Autodesk Inventor part; units mm, degrees
ref_plane "YZ Plane" through (0, 0, 0) normal (1, 0, 0) x (0, 1, 0)
ref_plane "XZ Plane" through (0, 0, 0) normal (0, 1, 0) x (-1, 0, 0)
ref_plane "XY Plane" through (0, 0, 0) normal (0, 0, 1) x (1, 0, 0)
sketch "Sketch3" plane through (0, 0, 0) normal (0, 0, 1) x (1, 0, 0)
  line L0 (-50, 45) -> (50, 45)
  line L1 (50, 45) -> (50, -45)
  line L2 (50, -45) -> (-50, -45)
  line L3 (-50, -45) -> (-50, 45)
  line L4 (-50, 45) -> (50, -45) construction
  line L5 (50, 45) -> (-50, -45) construction
  point P0 (0, 0)
  dimension "d4" = 100
  dimension "d5" = 90
extrude "Extrusion2" add sketch "Sketch3" along normal blind 4
sketch "Sketch4" plane through (0, 0, 4) normal (0, 0, 1) x (1, 0, 0)
  point P0 (0, 0)
sketch "Sketch5" plane through (0, 0, 4) normal (0, 0, 1) x (1, 0, 0)
  line L0 (50, 45) -> (-50, 45)
  line L1 (50, 45) -> (-50, 45)
  line L2 (-50, 45) -> (-50, 41)
  line L3 (-50, 41) -> (50, 41)
  line L4 (50, 41) -> (50, 45)
  point P0 (0, 0)
  dimension "d8" = 4
  dimension "d9" = 100
extrude "Extrusion3" add sketch "Sketch5" against normal blind 50
sketch "Sketch6" plane through (0, 0, 4) normal (0, 0, 1) x (1, 0, 0)
  line L0 (18, -31.18) -> (-18, -31.18)
  line L1 (-18, -31.18) -> (-18, 31.18)
  line L2 (-18, 31.18) -> (18, 31.18)
  line L3 (18, 31.18) -> (18, -31.18)
  line L4 (18, -31.18) -> (-18, 31.18) construction
  line L5 (-18, -31.18) -> (18, 31.18) construction
  circle A0 centre (-18, 31.18) radius 1.75
  circle A1 centre (18, 31.18) radius 1.75
  circle A2 centre (-18, -31.18) radius 1.75
  circle A3 centre (18, -31.18) radius 1.75
  point P0 (0, 0)
  dimension "d12" = 36
  dimension "d13" = 62.36
  dimension "d14" = 3.5
  dimension "d15" = 3.5
  dimension "d16" = 3.5
  dimension "d17" = 3.5
extrude "Extrusion4" cut sketch "Sketch6" against normal blind 50 contours A2 L1 L0 | L0 L1 A2 | A3 L3 L0 | L0 L3 A3 | A0 L2 L1 | L1 L2 A0 | A1 L2 L3 | L3 L2 A1
sketch "Sketch7" plane through (0, 0, 4) normal (0, 0, 1) x (1, 0, 0)
  line L0 (31.18, -18) -> (-31.18, -18)
  line L1 (-31.18, -18) -> (-31.18, 18)
  line L2 (-31.18, 18) -> (31.18, 18)
  line L3 (31.18, 18) -> (31.18, -18)
  line L4 (31.18, -18) -> (-31.18, 18) construction
  line L5 (-31.18, -18) -> (31.18, 18) construction
  circle A0 centre (-31.18, 18) radius 1.75
  circle A1 centre (31.18, 18) radius 1.75
  circle A2 centre (-31.18, -18) radius 1.75
  circle A3 centre (31.18, -18) radius 1.75
  point P0 (0, 0)
  dimension "d20" = 62.36
  dimension "d21" = 36
  dimension "d22" = 3.5
  dimension "d23" = 3.5
  dimension "d24" = 3.5
  dimension "d25" = 3.5
extrude "Extrusion5" cut sketch "Sketch7" against normal blind 50 contours A2 L1 L0 | L0 L1 A2 | A3 L3 L0 | L0 L3 A3 | A0 L2 L1 | L1 L2 A0 | A1 L2 L3 | L3 L2 A1
sketch "Sketch8" plane through (0, 0, 4) normal (0, 0, 1) x (1, 0, 0)
  circle A0 centre (0, 0) radius 25
  dimension "d28" = 50
extrude "Extrusion6" cut sketch "Sketch8" against normal blind 43.6625
sketch "Sketch9" plane through (-50, 45, 4) normal (0, 1, 0) x (1, 0, 0)
  line L0 (0, 50) -> (0, 0)
  line L1 (100, 0) -> (0, 0)
  line L2 (0, 0) -> (38, 0)
  line L3 (38, 0) -> (38, 7)
  line L4 (38, 7) -> (0, 7)
  line L5 (0, 7) -> (0, 0)
  circle A0 centre (38, 7) radius 1.75
  line L6 (0, 0) -> (38, 0)
  line L7 (38, 0) -> (38, 25)
  line L8 (38, 25) -> (0, 25)
  line L9 (0, 25) -> (0, 0)
  circle A1 centre (38, 25) radius 1.75
  point P0 (50, 4)
  dimension "d31" = 38
  dimension "d32" = 7
  dimension "d36" = 3.5
  dimension "d39" = 25
  dimension "d40" = 3.5
sketch "Sketch10" plane through (-50, 45, 4) normal (0, 1, 0) x (1, 0, 0)
  line L0 (100, 4) -> (100, 0)
  line L1 (100, 0) -> (0, 0)
  line L2 (100, 0) -> (62, 0)
  line L3 (62, 0) -> (62, 7)
  line L4 (62, 7) -> (100, 7)
  line L5 (100, 7) -> (100, 0)
  circle A0 centre (62, 7) radius 1.75
  line L6 (100, 0) -> (62, 0)
  line L7 (62, 0) -> (62, 25)
  line L8 (62, 25) -> (100, 25)
  line L9 (100, 25) -> (100, 0)
  line L10 (75, 0) -> (25, 0)
  circle A1 centre (62, 25) radius 1.75
  point P0 (50, 4)
  dimension "d33" = 38
  dimension "d34" = 7
  dimension "d35" = 3.5
  dimension "d37" = 25
  dimension "d38" = 3.5
sketch "Sketch11" plane through (-50, 45, 4) normal (0, 1, 0) x (1, 0, 0)
  point P0 (50, 4)
extrude "Extrusion7" cut sketch "Sketch9" against normal blind 43.6625 contours A1 L7 L8 | L8 L7 A1 | A0 L7 L4 | L4 L3 A0 | L7 A0 L3
extrude "Extrusion8" cut sketch "Sketch10" against normal blind 43.6625 contours A0 L3 L4 | L4 L7 A0 | L3 A0 L7 | A1 L7 L8 | L8 L7 A1
sketch "Sketch12" plane through (-50, 45, 4) normal (0, 1, 0) x (1, 0, 0)
  line L0 (0, 0) -> (100, 0)
  line L1 (0, 0) -> (10, 0)
  line L2 (10, 0) -> (10, 7)
  line L3 (10, 7) -> (0, 7)
  line L4 (0, 7) -> (0, 0)
  line L5 (100, 0) -> (0, 0)
  line L6 (0, 0) -> (10, 0)
  line L7 (10, 0) -> (10, 25)
  line L8 (10, 25) -> (0, 25)
  line L9 (0, 25) -> (0, 0)
  circle A0 centre (10, 7) radius 1.75
  circle A1 centre (10, 25) radius 1.75
  point P0 (50, 4)
  dimension "d45" = 10
  dimension "d46" = 7
  dimension "d47" = 25
  dimension "d48" = 3.5
  dimension "d49" = 3.5
extrude "Extrusion9" cut sketch "Sketch12" against normal blind 43.6625 contours A0 L3 L2 | L2 L7 A0 | A0 L7 L3 | A1 L7 L8 | L8 L7 A1
sketch "Sketch13" plane through (-50, 45, 4) normal (0, 1, 0) x (1, 0, 0)
  line L0 (0, 0) -> (100, 0)
  line L1 (100, 0) -> (90, 0)
  line L2 (90, 0) -> (90, 7)
  line L3 (90, 7) -> (100, 7)
  line L4 (100, 7) -> (100, 0)
  line L5 (100, 0) -> (90, 0)
  line L6 (90, 0) -> (90, 25)
  line L7 (90, 25) -> (100, 25)
  line L8 (100, 25) -> (100, 0)
  circle A0 centre (90, 25) radius 1.75
  circle A1 centre (90, 7) radius 1.75
  point P0 (50, 4)
  dimension "d52" = 10
  dimension "d53" = 7
  dimension "d54" = 25
  dimension "d55" = 3.5
  dimension "d56" = 3.5
extrude "Extrusion10" cut sketch "Sketch13" against normal blind 43.6625 contours A1 L6 L2 | L2 L3 A1 | L6 A1 L3 | A0 L7 L6 | L6 L7 A0
sketch "Sketch14" plane through (-50, 45, 4) normal (0, 1, 0) x (1, 0, 0)
  point P0 (50, 4)
sketch "Sketch15" plane through (-50, 45, 4) normal (0, 1, 0) x (1, 0, 0)
  line L0 (0, 50) -> (100, 50)
  line L1 (0, 50) -> (50, 50)
  line L2 (50, 50) -> (50, 42)
  line L3 (50, 42) -> (0, 42)
  line L4 (0, 42) -> (0, 50)
  line L5 (0, 50) -> (10, 50)
  line L6 (10, 50) -> (10, 42)
  line L7 (10, 42) -> (0, 42)
  line L8 (0, 42) -> (0, 50)
  line L9 (0, 4) -> (0, 50)
  line L10 (0, 50) -> (30, 50)
  line L11 (30, 50) -> (30, 42)
  line L12 (30, 42) -> (0, 42)
  line L13 (0, 42) -> (0, 50)
  line L14 (100, 4) -> (100, 50)
  line L15 (100, 50) -> (90, 50)
  line L16 (90, 50) -> (90, 42)
  line L17 (90, 42) -> (100, 42)
  line L18 (100, 42) -> (100, 50)
  line L19 (100, 50) -> (0, 50)
  line L20 (100, 50) -> (70, 50)
  line L21 (70, 50) -> (70, 42)
  line L22 (70, 42) -> (100, 42)
  line L23 (100, 42) -> (100, 50)
  circle A0 centre (50, 42) radius 1.75
  circle A1 centre (30, 42) radius 1.75
  circle A2 centre (10, 42) radius 1.75
  circle A3 centre (70, 42) radius 1.75
  circle A4 centre (90, 42) radius 1.75
  point P0 (50, 4)
  dimension "d59" = 50
  dimension "d60" = 8
  dimension "d61" = 10
  dimension "d62" = 30
  dimension "d63" = 10
  dimension "d64" = 30
  dimension "d65" = 3.5
  dimension "d66" = 3.5
  dimension "d67" = 3.5
  dimension "d68" = 3.5
  dimension "d69" = 3.5
extrude "Extrusion11" cut sketch "Sketch15" against normal blind 43.6625 contours A2 L3 L6 | L6 L3 A2 | L3 A2 | A1 L3 L11 | L11 L3 A1 | A0 L3 L2 | L2 L3 A0 | L3 A1 | A3 L22 L21 | L21 L22 A3 | A4 L17 L16 | L16 L22 A4 | L17 A4 L22
properties part number "ousterholderm600"
Could you check a few things on this model? Use its own coordinates, in mm. A direction names the side the tool comes from. Give positions to 0.01 mm unless a question says otherwise; leave off trailing zeros. Order: outer loops, then holes, each group sorted by start corner. A loop starts at its lowest first (then second) coordinate and runs counter-clockwise, first axis right, second up. Notation, with made-up numbers: (-1, 32.5) - (29, 32.5) arc R31 ccw to (29, 70.5) - close; hole circle Ø2 at (28.5, -40). An arc over 180 degrees is marked (long way). One line per item, written item: value. Start each with the question number.
1. Imagine slicing it at D-D on x = -15. List the corners of the cut face in (y, z) for me.
2. Imagine slicing it at B-B on z = -3. List the corners of the cut face in (x, y) for me, plus the area to 3 significant figures.
3. Thinking about a two-plate mould opening in X: for faces 1 (the face through (1, -45, 2)), 2 (the face through (-38.383, 43.028, -2.33)), 3 (the face through (50, 14, 1)), which applies, +X half, -X half, draft (parallel to the pull), parting line (faces both ways), or undercut?
4. Imagine slicing it at A-A on x = -40. List the corners of the cut face in (y, z) for me, plus the area to 3 significant figures.
5. If I drill on probe 1 along X at (y, z) = (31.18, 1.1); probe 2 along Z at (x, y) = (40, 43.85); probe 3 along X at (y, z) = (43, -38), over which ranges is the centre line in solid material (lowest first)?
6. For P1, Ø23, axis at x = 23, z = -24.5, coming from the -Y side; P2, Ø10, axis at y = -6, z = -4, coming from the -X side; P3, Ø2, axis at x = -12, z = -21, coming from the -Y side; P4, Ø4, axis at x = -31.18, y = 18, coming from the -Z side, each with a flat end and sliding along its axis, tell me the tip position at first contact or that it passes through.
7. For faces 4 (the face through (-1, 41, -23)), 5 (the face through (16.25, 31.26, 2.03)), which set-ups out of +Z, -Z, +X, -X, +Y, -Y let a thin tool reach every point of the face, with its end or its side?
8. Imagine slicing it at C-C on y = 0. List the corners of the cut face in (x, z) for me.
Values:
1. outline: (-45, 0) - (-20, 0) - (-20, 4) - (-45, 4) - close; (20, 0) - (41, 0) - (41, -46) - (45, -46) - (45, 4) - (20, 4) - close
2. outline: (-50, 41) - (-41.75, 41) - (-41.75, 45) - (-50, 45) - close; (-38.25, 41) - (-13.75, 41) - (-13.75, 45) - (-38.25, 45) - close; (-10.25, 41) - (10.25, 41) - (10.25, 45) - (-10.25, 45) - close; (13.75, 41) - (38.25, 41) - (38.25, 45) - (13.75, 45) - close; (41.75, 41) - (50, 41) - (50, 45) - (41.75, 45) - close
2. area: 344 mm²
3. face 1: draft
3. face 2: undercut
3. face 3: +X half
4. outline: (-45, 0) - (41, 0) - (41, -1.25) - (45, -1.25) - (45, 4) - (-45, 4) - close; (41, -46) - (45, -46) - (45, -39.75) - (41, -39.75) - close; (41, -36.25) - (45, -36.25) - (45, -22.75) - (41, -22.75) - close; (41, -19.25) - (45, -19.25) - (45, -4.75) - (41, -4.75) - close
4. area: 502 mm²
5. probe 1: -50 to -19.75, -16.25 to 16.25, 19.75 to 50
5. probe 2: -46 to -39.75, -36.25 to -22.75, -19.25 to -4.75, -1.25 to 4
5. probe 3: -50 to -41.75, -38.25 to -21.75, -18.25 to -1.75, 1.75 to 18.25, 21.75 to 38.25, 41.75 to 50
6. P1: y = 41
6. P2: x = -50
6. P3: through
6. P4: z = 0
7. face 4: -Z, +X, -X, -Y
7. face 5: +Z, -Z
8. outline: (-50, 0) - (-25, 0) - (-25, 4) - (-50, 4) - close; (25, 0) - (50, 0) - (50, 4) - (25, 4) - close
